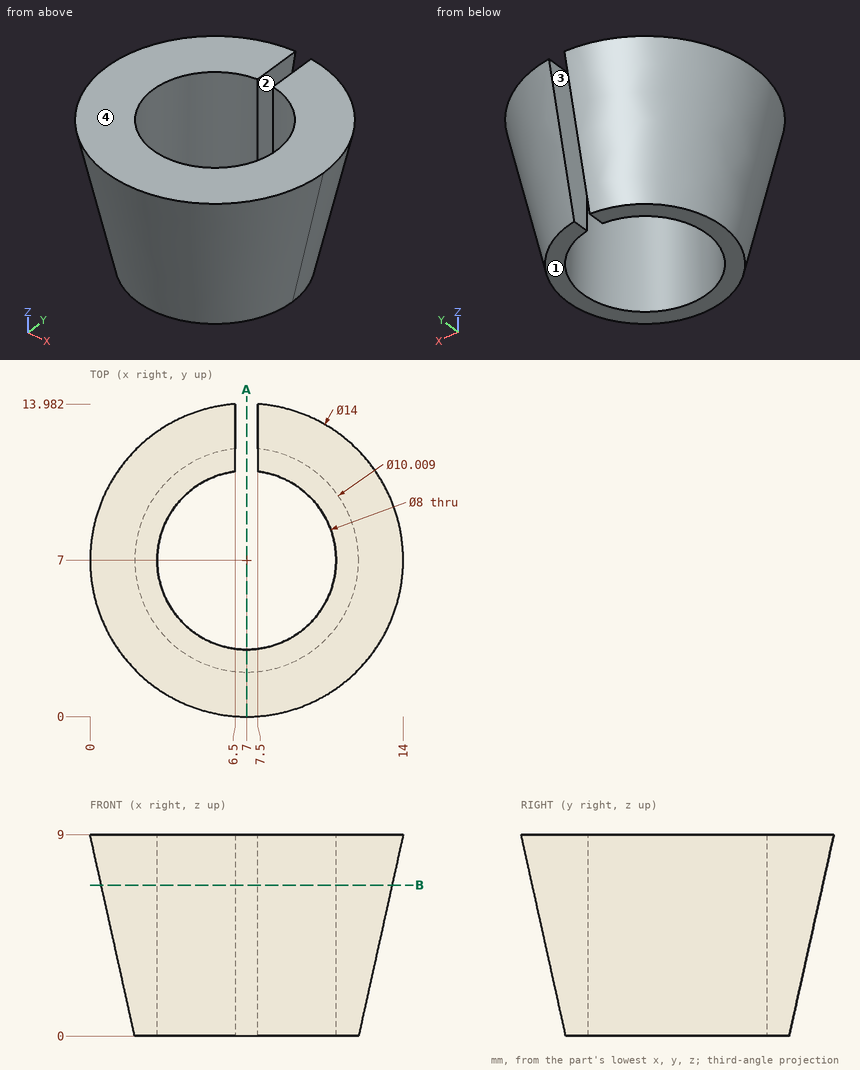
Design review of the part shown in the three views and the two pictorial views. Dimensions are in mm from the part's minimum x, y and z. A direction names the side the tool comes from. Give positions to 0.01 mm unless a question says otherwise; leave off trailing zeros. Loops run counter-clockwise (first coordinate to the right, second up) from the corner with the lowest first, then second, coordinate; pieces in that order, holes last. Notation, with made-up numbers: (21.25, 7) -> (80.25, 7) arc R15 cw to (80.25, 30) -> close; hole circle Ø9 at (-8.75, 52). An arc over 180 degrees is marked (long way). Answer as a JSON object with one key per item and string values. Group by question number.
Q1. Take a section at A-A (x = 7). Write out the cut boundary in (y, z) (1 decimal), plus the area to 3 significant figures.
Q2. Wall thickness on line 1 along X through (y, z) = (7, 5.75); line 2 along X through (y, z) = (7, 4.75); line 3 along Y through (x, z) = (9, 2.25) (1 decimal): over which ranges is each line inside the solid? List them lowest first.
Q3. Take a section at B-B (z = 6.75). Write out the cut boundary in (x, y).
Q4. Insertion check: pin 1 (3 mm diameter, centred on y = 7.5, z = 4, fed in from -X) (1 decimal); pin 2 (3.5 mm diameter, centred on y = 13, z = 5, fed in from +X); pin 3 (2.5 mm diameter, centred on y = 13, z = 2.5, fed in from -X) (1 decimal). Each pin has a flat end and moves straight along its axis. Give the tip position at first contact, or say it passes through.
Q5. Tool access review of the marked faces 1 and 2: name each direction out of +Z, -Z, +X, -X, +Y, -Y from which nothing blocks a thin tool from reaching the whole face with its end or side.
Q6. Draft analysis for pull direction X (two halves, no side actions). For the marked faces 3 and 4, state which applies: pulls with the +X half, pulls with the -X half, needs draft (parallel to the pull), parting line crosses it, or undercut.
Answer below:
{
 "1": {"outline": "(0, 9) -> (2, 0) -> (3, 0) -> (3, 9) -> close", "area": "18.0 mm2"},
 "2": {"line 1": "x = 0.72 to 3, 11 to 13.28", "line 2": "x = 0.94 to 3, 11 to 13.06", "line 3": "y = 1.9 to 3.5, 10.5 to 12.1"},
 "3": {"outline": "(6.5, 10.97) -> (6.5, 13.48) arc R6.5 ccw (long way) to (7.5, 13.48) -> (7.5, 10.97) arc R4 cw (long way) to start"},
 "4": {"pin 1": "stops at x = 0.8", "pin 2": "stops at x = 11.48", "pin 3": "stops at x = 4"},
 "5": {"face 1": "-Z, +X, -X, +Y, -Y", "face 2": "+Z, -Z, +Y"},
 "6": {"face 3": "undercut", "face 4": "needs draft"}
}
